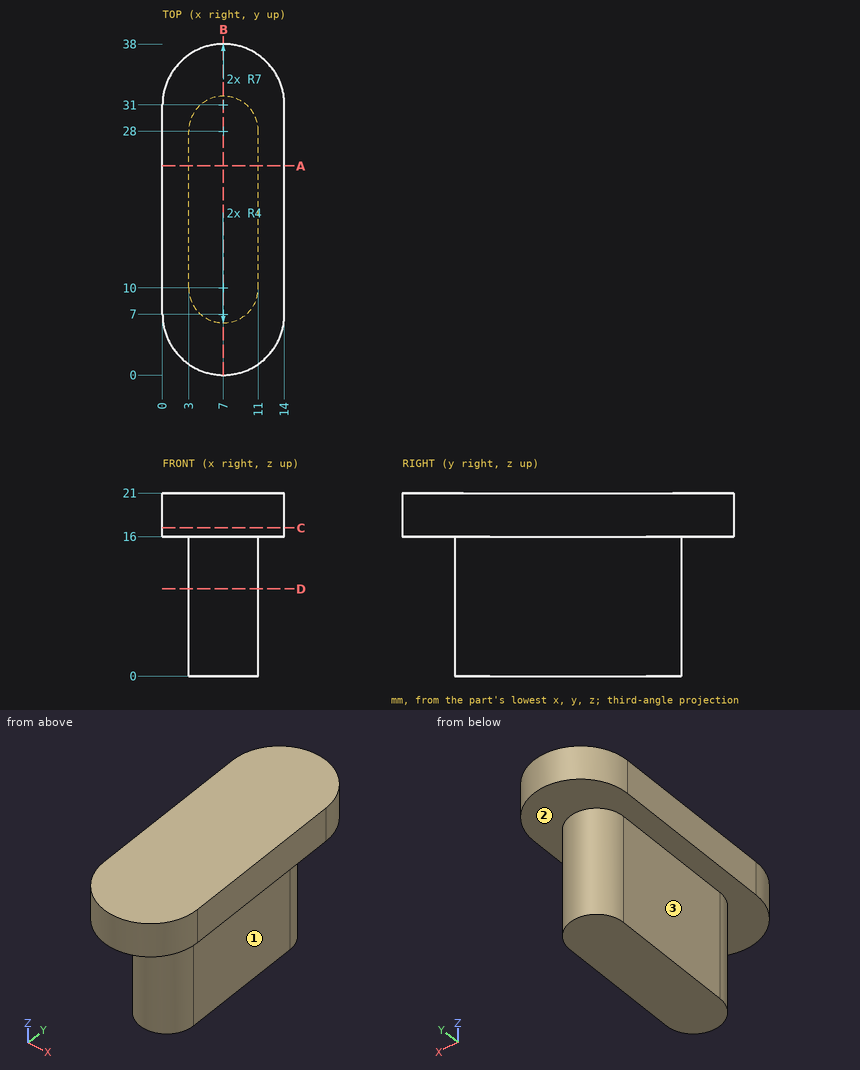
Job drawing, mm, ordinate dimensions from the low corner. One solid piece. A direction names the side the tool comes from. Give positions to 0.01 mm unless a question says otherwise; leave off trailing zeros. Write each loop counter-clockwise with the first axis right and the second up, starting at its lowest first coordinate (ties: lowest second). Pieces come first, ordered by that corner, then holes. Notation, with made-up numbers: (27.25, 74) -> (56.25, 74) arc R18 ccw to (56.25, 84) -> close; hole circle Ø9 at (-34, 53). An arc over 180 degrees is marked (long way). Return JSON: item names as keys, results as strings.
Item 1: Tool access for the marked faces 1, 2 and 3: list every direction of +Z, -Z, +X, -X, +Y, -Y with a clear straight run to the whole face (end or side of a thin tool).
Answer below:
{"face 1": "-Z, +X, +Y, -Y", "face 2": "-Z", "face 3": "-Z, -X, +Y, -Y"}
Item 2: Band-saw the part on D-D (z = 10). List the corners of the cut face in (x, y).
Answer below:
{"outline": "(3, 10) arc R4 ccw to (11, 10) -> (11, 28) arc R4 ccw to (3, 28) -> close"}
Item 3: Band-saw the part on B-B (x = 7). List the corners of the cut face in (y, z), then the cut area to 3 significant figures.
Answer below:
{"outline": "(0, 16) -> (6, 16) -> (6, 0) -> (32, 0) -> (32, 16) -> (38, 16) -> (38, 21) -> (0, 21) -> close", "area": "606 mm2"}
Item 4: Band-saw the part on A-A (y = 24). List the corners of the cut face in (x, z).
Answer below:
{"outline": "(0, 16) -> (3, 16) -> (3, 0) -> (11, 0) -> (11, 16) -> (14, 16) -> (14, 21) -> (0, 21) -> close"}
Item 5: Drill centre lines: probe 1 along X at (y, z) = (27.5, 15); probe 2 along Z at (x, y) = (2.5, 14.5); probe 3 along Y at (x, z) = (4.5, 2.5). Where is each one in solid material? Low to high.
Answer below:
{"probe 1": "x = 3 to 11", "probe 2": "z = 16 to 21", "probe 3": "y = 6.88 to 31.12"}
Item 6: Drop flat-ended pins along their axis: pin 1 (3 mm diameter, centred on y = 17.5, z = 5.5, fed in from -X); pin 2 (6 mm diameter, centred on x = 8.5, z = 7.5, fed in from -Y); pin 3 (6 mm diameter, centred on x = 5, z = 11, fed in from +Y). Give the stop position or say it passes through.
Answer below:
{"pin 1": "stops at x = 3", "pin 2": "stops at y = 6", "pin 3": "stops at y = 32"}
Item 7: Band-saw the part on C-C (z = 17). List the corners of the cut face in (x, y).
Answer below:
{"outline": "(0, 7) arc R7 ccw to (14, 7) -> (14, 31) arc R7 ccw to (0, 31) -> close"}
